Autodesk Inventor part; units mm, degrees
ref_plane "YZ Plane" through (0, 0, 0) normal (1, 0, 0) x (0, 1, 0)
ref_plane "XZ Plane" through (0, 0, 0) normal (0, 1, 0) x (-1, 0, 0)
ref_plane "XY Plane" through (0, 0, 0) normal (0, 0, 1) x (1, 0, 0)
sketch "Sketch1" plane through (0, 0, 0) normal (0, 1, 0) x (-1, 0, 0)
  line L0 (15, 0) -> (15, -15)
  line L1 (15, -15) -> (0, -15)
  line L2 (0, -15) -> (0, -12)
  line L3 (0, -12) -> (12, -12)
  line L4 (12, -12) -> (12, 0)
  line L5 (12, 0) -> (15, 0)
  point P0 (0, 0)
  dimension "d0" = 15
  dimension "d1" = 15
  dimension "d10" = 3
  dimension "d11" = 12
  dimension "d12" = 12
extrude "Extrusion1" add sketch "Sketch1" along normal blind 86
sketch "Sketch4" plane through (-12, 0, 0) normal (1, 0, 0) x (0, 0, -1)
  line L0 (0, 0) -> (0, 86)
  line L1 (12, 0) -> (12, 86)
  line L2 (0, 86) -> (12, 86)
  line L3 (12, 86) -> (12, 83)
  line L4 (12, 83) -> (0, 83)
  line L5 (0, 83) -> (0, 86)
  dimension "d13" = 3
extrude "Extrusion3" add sketch "Sketch4" along normal blind 3
sketch "Sketch6" plane through (-12, 0, -12) normal (0, 0, 1) x (1, 0, 0)
  line L0 (3, 86) -> (12, 86)
  line L1 (12, 86) -> (3, 86)
  line L2 (3, 86) -> (3, 83)
  line L3 (3, 83) -> (12, 83)
  line L4 (12, 83) -> (12, 86)
  point P0 (12, 0)
extrude "Extrusion4" add sketch "Sketch6" along normal blind 12
fillet "Fillet3" radius 2 7 edges at (-7.5, 86, -15) (-15, 86, -7.5) (-15, 43, -15) (0, 43, -15) (-7.5, 86, 0) (0, 86, -7.5) (-15, 43, 0)
sketch "Sketch11" plane through (0, 86, 0) normal (0, 1, 0) x (1, 0, 0)
  arc A0 (-15, 2) -> (-13, 0) centre (-13, 2) ccw
  line L0 (0, 10.8348) -> (0, 14)
  line L1 (-9, 9) -> (0, 9)
  line L2 (0, 9) -> (0, 10.8348)
  line L3 (-9, 15) -> (0, 15)
  line L4 (0, 15) -> (0, 9)
  line L5 (-9, 15) -> (-9, 9)
  line L6 (0, 0) -> (0, 13)
  point P0 (-13, 0)
  point P1 (0, 15)
extrude "Extrusion7" cut sketch "Sketch11" against normal blind 6.5
sketch "Sketch12" plane through (-12, 0, -12) normal (0, 0, 1) x (1, 0, 0)
  line L0 (12, 33) -> (21, 33) construction
  line L1 (12, 0) -> (12, 79.5)
  line L2 (3, 36) -> (3, 35.5)
  line L3 (12, 38.5) -> (3, 38.5)
  line L4 (3, 38.5) -> (3, 35)
  line L5 (3, 35) -> (12, 35)
  dimension "d44" = 3.5
  dimension "d45" = 9
extrude "Extrusion8" cut sketch "Sketch12" against normal through all
properties part number "DoosjeHoeken" material "ABS Plastic"
Source: CAD feature listing. Evaluate the final solid. Frame: model axes, mm. A direction names the side the tool comes from. Coordinates: 2 decimals unless noted, no trailing zeros. Write each loop counter-clockwise with the first axis right and the second up, starting at its lowest first coordinate (ties: lowest second). Pieces come first, ordered by that corner, then holes. Notation, with made-up numbers: M 27.5,36 L 83.5,36 A24 ccw 83.5,48 Z; hole C -26,38 d7. An arc over 180 degrees is marked long. Use a Markdown table: item, result.
1) Section C-C, the plane z = -9.75. Output: boundary loops of the cut face in (x, y), then the cut area to 3 significant figures.
Conclusion:
| item | result |
|---|---|
| outline | M -15,0 L -12,0 L -12,83 L -9,83 L -9,86 L -13,86 A2 ccw -15,84 Z |
| area | 266 mm^2 |
2) Section A-A, the plane x = -6. Output: boundary loops of the cut face in (y, z), then the cut area to 3 significant figures.
Conclusion:
| item | result |
|---|---|
| outline | M 0,-15 L 35,-15 L 35,-12 L 0,-12 Z; M 38.5,-15 L 79.5,-15 L 79.5,-12 L 38.5,-12 Z; M 83,-9 L 86,-9 L 86,-2 A2 ccw 84,0 L 83,0 Z |
| area | 254 mm^2 |
3) Mould query, pull axis Y, two halves, no side actions, for faces 6 (the flat face through (-4, 38.5, -13)), 7 (the flat face through (-8, 86, -6)), 8 (the flat face through (-9, 37, -13)), 9 (the flat face through (-10.7, 0, -12.4)). Classes: pulls with the +Y half, pulls with the -Y half, needs draft (parallel to the pull), parting line crosses it, or undercut.
Conclusion:
| item | result |
|---|---|
| face 6 | undercut |
| face 7 | pulls with the +Y half |
| face 8 | undercut |
| face 9 | pulls with the -Y half |
4) Section D-D, the plane x = -11. Output: boundary loops of the cut face in (y, z).
Conclusion:
| item | result |
|---|---|
| outline | M 0,-15 L 84,-15 A2 ccw 86,-13 L 86,-2 A2 ccw 84,0 L 83,0 L 83,-12 L 0,-12 Z |
5) Reachability of faces 1 (the flat face through (-5, 85, -9)), 2 (the flat face through (-12, 41, -6)), 3 (the flat face through (-5, 79.5, -14)), 4 (the cylindrical face through (-10.97, 85.4, -14.43)), 5 (the flat face through (-9, 84, -13)) from +Z, -Z, +X, -X, +Y, -Y: full face, straight path, thin tool, end or side. Return the list, or none.
Conclusion:
| item | result |
|---|---|
| face 1 | -Z, +X, +Y, -Y |
| face 2 | +Z, +X, -Y |
| face 3 | +Z, -Z, +X, +Y |
| face 4 | -Z, +X, -X, +Y |
| face 5 | -Z, +X, +Y |
6) First-contact query: pin 1 Ø3.5 at (x, z) = (-6, -13.5) entering from +Y; pin 2 Ø0.9 at (x, y) = (-4.5, 84) entering from -Z; pin 3 Ø1.5 at (y, z) = (36, -13) entering from +X. Flat tips, straight axial feed; report the tip coordinate or a pass-through.
Conclusion:
| item | result |
|---|---|
| pin 1 | stops at y = 79.5 |
| pin 2 | stops at z = -9 |
| pin 3 | stops at x = -9 |
7) Section B-B, the plane y = 80.5. Output: boundary loops of the cut face in (x, z), then the cut area to 3 significant figures.
Conclusion:
| item | result |
|---|---|
| outline | M -15,-13 A2 ccw -13,-15 L -9,-15 L -9,-12 L -12,-12 L -12,0 L -13,0 A2 ccw -15,-2 Z |
| area | 52.3 mm^2 |
8) Ray query, L1, parallel to Y at x = -8, z = -2.25; L2, parallel to Z at x = -7.75, y = 20.5. Return the intervals inside material, ascending.
Conclusion:
| item | result |
|---|---|
| L1 | y = 83 to 86 |
| L2 | z = -15 to -12 |
